The listing builds one solid part. Answer for the finished solid, in the listing's coordinates (mm). A direction names the side the tool comes from. Round coordinates to 2 decimals unless told otherwise and drop trailing zeros. Write each loop counter-clockwise with the first axis right and the second up, starting at its lowest first coordinate (ties: lowest second). Pieces come first, ordered by that corner, then holes.
Item 1: A tool of negligible diameter and unlimited length cuts with its end or side. For faces 1 (the face through (51.43, 4.93, 62.18)), 2 (the face through (181, -84, -85)), from which of +Z, -Z, +X, -X, +Y, -Y can it reach the whole face along a straight path? Write none if from no direction.
Item 2: For a pull along Y with two mould halves and no side action, classify faces 3 (the face through (356, -65, -20)), 4 (the face through (19.447, -154.214, -90.07)), 5 (the face through (181, 0, 1)), 6 (the face through (341.754, -150.187, -90.07)) as +Y half, -Y half, draft (parallel to the pull), parting line (faces both ways), or undercut.
Item 3: Find section B-B on x = 277.5. Give the vertices of the cut face in (y, z), then the cut area to 3 significant figures.
Item 4: Each of these flat-tipped pins is pushed along its axis until it touches: pin 1 (7 mm diameter, centred on x = 20, y = -150, fed in from -Z); pin 2 (10 mm diameter, centred on x = 20, y = -10, fed in from +Z); pin 3 (12 mm diameter, centred on x = 141, z = 29, fed in from -Y). Where does it stop, or does it pass through?
Item 5: Find section C-C on z = 54. Give the vertices of the cut face in (x, y), then the cut area to 3 significant figures.
Item 6: Find the intervals of material crossed by probe 1 along X at (y, z) = (-150, -87.5); probe 2 along Y at (x, z) = (20, -88.25); probe 3 along Z at (x, y) = (52.5, 5), in increasing order.
Item 7: Find section A-A on y = -10. Give the vertices of the cut face in (x, z).
Item 8: Find section D-D on z = -33. Give the vertices of the cut face in (x, y), then the cut area to 3 significant figures.
```python
from build123d import *

# Parameters (mm, degrees)
F1_DEPTH  = 366
F2_R      = 8.25
F3_DEPTH  = 10.001
F4_W      = 10
F4_H      = 170
F5_DEPTH  = 170
F8_DEPTH  = 366.001
F9_R      = 4.25
F10_DEPTH = 180.001


with BuildPart() as f1:
    # F0 (on Right) → F1 (new body)
    with BuildSketch(Plane.YZ):
        Polygon((10, -95), (10, 85), (0, 85), (0, -85), (-170, -85), (-170, -95), align=None)
    extrude(amount=F1_DEPTH)

    # F2 (on face) → F3 (cut, through all)
    with BuildSketch(Plane.XZ):
        with Locations((52.5, 54)):
            Circle(F2_R)
        with Locations((277.5, 54)):
            Circle(F2_R)
        with Locations((277.5, -64)):
            Circle(F2_R)
        with Locations((52.5, -64)):
            Circle(F2_R)
    extrude(amount=-F3_DEPTH, mode=Mode.SUBTRACT)

    # F4 (on face) → F5 (join)
    with BuildSketch(Plane.XZ):
        with Locations((5, 0)):
            Rectangle(F4_W, F4_H)
        with Locations((361, 0)):
            Rectangle(F4_W, F4_H)
    extrude(amount=F5_DEPTH)

    # F7 (on face) + F6 (on face) → F8 (cut, through all)
    with BuildSketch(Plane(origin=(0, 0, 0), x_dir=(0, -1, 0), z_dir=(-1, 0, 0))):
        Polygon((170, 85), (0, 85), (170, -85), align=None)
    with BuildSketch(Plane.YZ.offset(366)):
        Polygon((-170, -85), (5, 85), (-170, 85), align=None)
    extrude(amount=-F8_DEPTH, dir=(-1, 0, 0), mode=Mode.SUBTRACT)

    # F9 (on face) → F10 (cut, through all)
    with BuildSketch(Plane(origin=(0, 0, -95), x_dir=(1, 0, 0), z_dir=(0, 0, -1))):
        with Locations((20, 150)):
            Circle(F9_R)
        with Locations((20, 10)):
            Circle(F9_R)
        with Locations((346, 10)):
            Circle(F9_R)
        with Locations((346, 150)):
            Circle(F9_R)
    extrude(amount=-F10_DEPTH, mode=Mode.SUBTRACT)


solid = f1.part
```
Check values:
1. face 1: +Y, -Y
1. face 2: +Z, -Y
2. face 3: draft
2. face 4: undercut
2. face 5: -Y half
2. face 6: undercut
3. outline: (-170, -95) - (10, -95) - (10, -72.25) - (0, -72.25) - (0, -85) - (-170, -85) - close; (0, -55.75) - (10, -55.75) - (10, 45.75) - (0, 45.75) - close; (0, 62.25) - (10, 62.25) - (10, 85) - (0, 85) - close
3. area: 3,170 mm2
4. pin 1: passes through
4. pin 2: stops at z = -85
4. pin 3: stops at y = 0
5. outline: (0, -31) - (10, -31) - (10, 0) - (44.25, 0) - (44.25, 10) - (0, 10) - close; (60.75, 0) - (269.25, 0) - (269.25, 10) - (60.75, 10) - close; (285.75, 0) - (356, 0) - (356, -31) - (366, -31) - (366, 10) - (285.75, 10) - close
5. area: 3,950 mm2
6. probe 1: x = 0 to 15.75, 24.25 to 341.75, 350.25 to 366
6. probe 2: y = -170 to -154.25, -145.75 to -14.25, -5.75 to 10
6. probe 3: z = -95 to -72.25, -55.75 to 45.75, 62.25 to 85
7. outline: (0, -95) - (15.75, -95) - (15.75, -85) - (10, -85) - (10, 75) - (0, 75) - close; (24.25, -95) - (341.75, -95) - (341.75, -85) - (24.25, -85) - close; (350.25, -95) - (366, -95) - (366, 75) - (356, 75) - (356, -85) - (350.25, -85) - close
8. outline: (0, -118) - (10, -118) - (10, 0) - (356, 0) - (356, -118) - (366, -118) - (366, 10) - (0, 10) - close
8. area: 6,020 mm2
